Here's how the part is built. I have some questions about the finished solid (model axes, mm). Face numbers are marked on the shaded views. A direction names the side the tool comes from. Coordinates: 2 decimals unless noted, no trailing zeros. Loops run counter-clockwise (first coordinate to the right, second up) from the corner with the lowest first, then second, coordinate; pieces in that order, holes last. Notation, with made-up numbers: (-28, 12.25) -> (16, 12.25) arc R24 ccw to (16, 40.25) -> close; hole circle Ø7 at (-38.5, 52). An arc over 180 degrees is marked (long way). Answer as a JSON object with one key per item and string values. Group by question number.
Q1. I want a section at A-A on z = 0. Write out the boundary of the cut face in (x, y).
Q2. I'm going to push flat-ended pins straight in: pin 1 (4 mm diameter, centred on y = 4, z = -0.5, fed in from -X); pin 2 (6 mm diameter, centred on x = 18, y = 6.5, fed in from +Z); pin 3 (3 mm diameter, centred on x = 26.5, y = 3.5, fed in from -Z); pin 4 (8 mm diameter, centred on x = 19, y = 1, fed in from +Z). Where does each tip first touch, or does it pass through?
Q3. On a 3-axis mill with a long thin cutter (end or side, diameter ignored), from which of +Z, -Z, +X, -X, +Y, -Y can I reach the whole of each face in a straight line? I mean the marked faces 1 and 2. Say none if no direction works.
Q4. I need wall thicknesses on line 1 (X direction, y = 0.25, z = 4.25); line 2 (X direction, y = -5.75, z = 5.75); line 3 (Y direction, x = 34, z = -3.25). Which ranges of each line are inside material? Lowest first, please.
Q5. I want a section at C-C on x = 13.5. Write out the boundary of the cut face in (y, z).
```python
from build123d import *

# Parameters (mm, degrees)
SCHIZZO1_R                   = 10
ESTRUSIONE_ESTRUSIONE1_DEPTH = 3
SCHIZZO2_R                   = 6
ESTRUSIONE_ESTRUSIONE2_DEPTH = 35
SCHIZZO3_W                   = 1.05
SCHIZZO3_H                   = 2
SMUSSO1_SIZE                 = 1
SMUSSO2_SIZE                 = 0.5
RACCORDO1_R                  = 0.5


with BuildPart() as part:
    # Schizzo1 → Estrusione-Estrusione1 (new body)
    with BuildSketch(Plane(origin=(0, 0, 0), x_dir=(0, 0, -1), z_dir=(1, 0, 0))):
        Circle(SCHIZZO1_R)
    extrude(amount=ESTRUSIONE_ESTRUSIONE1_DEPTH)

    # Schizzo2 → Estrusione-Estrusione2 (add)
    with BuildSketch(Plane(origin=(3, 0, 0), x_dir=(0, 0, -1), z_dir=(1, 0, 0))):
        Circle(SCHIZZO2_R)
    extrude(amount=ESTRUSIONE_ESTRUSIONE2_DEPTH)

    # Schizzo3 → Taglia-Rivoluzione1 (revolve, cut)
    with BuildSketch(Plane.XY, mode=Mode.PRIVATE) as taglia_rivoluzione1_sk:
        with Locations((34.475, 5)):
            Rectangle(SCHIZZO3_W, SCHIZZO3_H)
    revolve(taglia_rivoluzione1_sk.sketch.rotate(Axis((0, 0, 0), (1, 0, 0)), 90), axis=Axis((0, 0, 0), (1, 0, 0)), mode=Mode.SUBTRACT)

    # Smusso1
    smusso1_edges = [part.edges().sort_by_distance(p)[0] for p in [
        (38, 0, 6),
    ]]
    chamfer(smusso1_edges, length=SMUSSO1_SIZE)

    # Smusso2
    smusso2_edges = [part.edges().sort_by_distance(p)[0] for p in [
        (0, 0, 10),
        (3, 0, 10),
    ]]
    chamfer(smusso2_edges, length=SMUSSO2_SIZE)

    # Raccordo1
    raccordo1_edges = [part.edges().sort_by_distance(p)[0] for p in [
        (3, 0, 6),
    ]]
    fillet(raccordo1_edges, radius=RACCORDO1_R)


solid = part.part
```
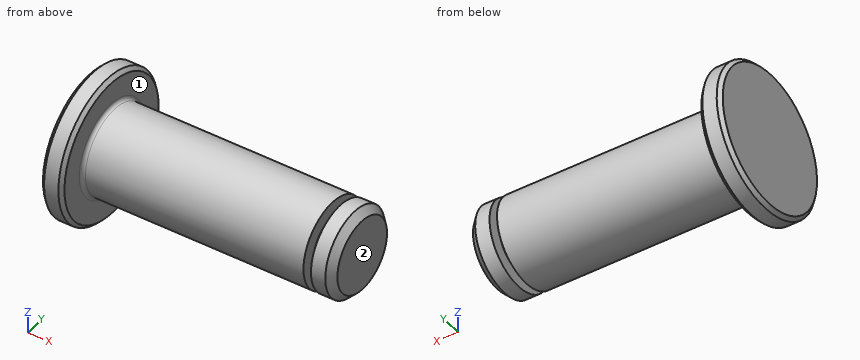
Result set:
{
 "1": {"outline": "(0, -9.5) -> (0.5, -10) -> (2.5, -10) -> (3, -9.5) -> (3, -6.5) arc R0.5 cw to (3.5, -6) -> (33.95, -6) -> (33.95, -4) -> (35, -4) -> (35, -6) -> (37, -6) -> (38, -5) -> (38, 5) -> (37, 6) -> (35, 6) -> (35, 4) -> (33.95, 4) -> (33.95, 6) -> (3.5, 6) arc R0.5 cw to (3, 6.5) -> (3, 9.5) -> (2.5, 10) -> (0.5, 10) -> (0, 9.5) -> close"},
 "2": {"pin 1": "stops at x = 0", "pin 2": "stops at z = 4.87", "pin 3": "stops at z = -5.66", "pin 4": "stops at z = 6"},
 "3": {"face 1": "+X", "face 2": "+Z, -Z, +X, +Y, -Y"},
 "4": {"line 1": "x = 0 to 33.95, 35 to 38", "line 2": "x = 0 to 3", "line 3": "y = -2.33 to 2.33"},
 "5": {"outline": "circle Ø12 at (0, 0)"}
}
